from build123d import *

# Parameters (mm, degrees)
SKETCH1_W           = 24
SKETCH1_H           = 40
SKETCH2_W           = 20
SKETCH2_H           = 30
SKETCH3_W           = 20
SKETCH3_H           = 30
SKETCH4_W           = 16
SKETCH4_H           = 16
SKETCH5_W           = 11.6
SKETCH5_H           = 11.6
BOSS_EXTRUDE1_DEPTH = 10
SKETCH6_R           = 2.3
CUT_EXTRUDE1_DEPTH  = 6
SKETCH7_R           = 2.3
CUT_EXTRUDE2_DEPTH  = 6
FILLET1_R           = 1
SKETCH8_W           = 8.4
SKETCH8_H           = 24.4
CUT_EXTRUDE3_DEPTH  = 20
SKETCH9_R           = 2.3
CUT_EXTRUDE4_DEPTH  = 6


with BuildPart() as part:
    # Sketch1 → Loft1 section 0
    with BuildSketch(Plane(origin=(0, 0, 0), x_dir=(1, 0, 0), z_dir=(0, 1, 0))):
        Rectangle(SKETCH1_W, SKETCH1_H)
    # Sketch2 → Loft1 section 1
    with BuildSketch(Plane(origin=(0, 50, 0), x_dir=(1, 0, 0), z_dir=(0, 1, 0))):
        Rectangle(SKETCH2_W, SKETCH2_H)
    loft()

    # Sketch3 → Loft2 section 0
    with BuildSketch(Plane(origin=(0, 50, 0), x_dir=(1, 0, 0), z_dir=(0, 1, 0))):
        Rectangle(SKETCH3_W, SKETCH3_H)
    # Sketch4 → Loft2 section 1
    with BuildSketch(Plane(origin=(0, 76, 0), x_dir=(1, 0, 0), z_dir=(0, 1, 0))):
        Rectangle(SKETCH4_W, SKETCH4_H)
    loft()

    # Sketch5 → Boss-Extrude1 (add)
    with BuildSketch(Plane(origin=(0, 76, 0), x_dir=(1, 0, 0), z_dir=(0, 1, 0))):
        Rectangle(SKETCH5_W, SKETCH5_H)
    extrude(amount=BOSS_EXTRUDE1_DEPTH)

    # Sketch6 → Cut-Extrude1 (cut)
    with BuildSketch(Plane.XY.offset(5.8)):
        with Locations((-3, 80)):
            Circle(SKETCH6_R)
    extrude(amount=-CUT_EXTRUDE1_DEPTH, mode=Mode.SUBTRACT)

    # Sketch7 → Cut-Extrude2 (cut)
    with BuildSketch(Plane(origin=(0, 0, -5.8), x_dir=(-1, 0, 0), z_dir=(0, 0, -1))):
        with Locations((-3, 80)):
            Circle(SKETCH7_R)
    extrude(amount=-CUT_EXTRUDE2_DEPTH, mode=Mode.SUBTRACT)

    # Fillet1
    fillet1_edges = [part.edges().sort_by_distance(p)[0] for p in [
        (0, 86, 5.8),
        (5.8, 86, 0),
        (0, 86, -5.8),
        (-5.8, 86, 0),
    ]]
    fillet(fillet1_edges, radius=FILLET1_R)

    # Sketch8 → Cut-Extrude3 (cut)
    with BuildSketch(Plane.XZ):
        Rectangle(SKETCH8_W, SKETCH8_H)
    extrude(amount=-CUT_EXTRUDE3_DEPTH, mode=Mode.SUBTRACT)

    # Sketch9 → Cut-Extrude4 (cut)
    with BuildSketch(Plane.XZ):
        with Locations((0, 16)):
            Circle(SKETCH9_R)
        with Locations((0, -16)):
            Circle(SKETCH9_R)
    extrude(amount=-CUT_EXTRUDE4_DEPTH, mode=Mode.SUBTRACT)


solid = part.part
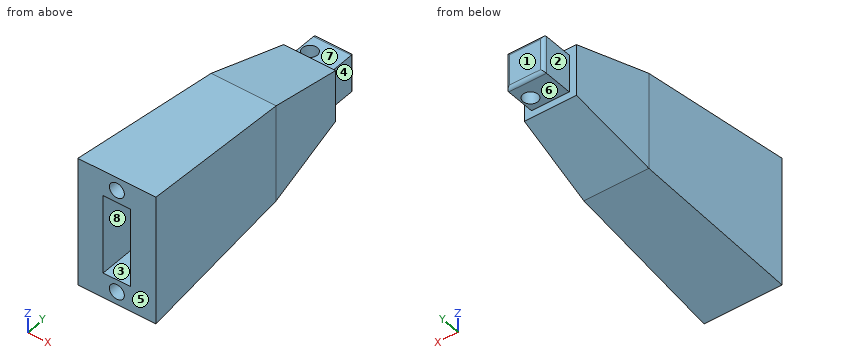
CAD build for the part. Positions are in the model's coordinates, mm. Face numbers are marked on the shaded views. A direction names the side the tool comes from. Coordinates: 2 decimals unless noted, no trailing zeros. Loops run counter-clockwise (first coordinate to the right, second up) from the corner with the lowest first, then second, coordinate; pieces in that order, holes last. Notation, with made-up numbers: (28.25, 4.5) - (40.25, 4.5) arc R12 ccw to (40.25, 10.5) - close; hole circle Ø8 at (36, 82.25). An arc over 180 degrees is marked (long way). Write item = value, one per line. Start each with the question number.
Q1. Which spindle directions (+Z, -Z, +X, -X, +Y, -Y) get a long thin tool onto all of the face, cutting with end or side? Do the marked faces 4, 5, 6, 7 and 8. Say none if no direction does.
Q2. Flat gauge pins, fed straight in: pin 1 Ø2.5 at (x, z) = (2, -5) entering from -Y; pin 2 Ø1.4 at (x, y) = (-2, 79.5) entering from +Z; pin 3 Ø4 at (x, y) = (4.5, 36.5) entering from +Z. Where does each tip first touch, or does it go through?
Q3. Cut at A-A, the plane y = 80. List the corners of the cut face in (x, z), then the cut area to 3 significant figures.
Q4. Pull direction X, two halves, no side cores. Call the marked faces 1, 2 and 3: pulls with the +X half, pulls with the -X half, needs draft (parallel to the pull), parting line crosses it, or undercut.
Q5. Drill centre lines: L1, parallel to Y at x = 3, z = -3.5; L2, parallel to Y at x = 7.25, z = -3.5; L3, parallel to Z at x = -2.5, y = 79. Where is each one in solid material? Low to high.
Computed:
q1.face_4 = +Z, -Z, +X, +Y
q1.face_5 = +Z, -Z, +X, -X, -Y
q1.face_6 = -Z, +X, -X, +Y
q1.face_7 = +Z, +X, -X, +Y
q1.face_8 = -Y
q2.pin_1 = 20
q2.pin_2 = -0.2
q2.pin_3 = 16.55
q3.outline = (-5.8, -5.8) - (0.7, -5.8) - (0.7, 0.2) - (5.3, 0.2) - (5.3, -5.8) - (5.8, -5.8) - (5.8, 5.8) - (-0.7, 5.8) - (-0.7, -0.2) - (-5.3, -0.2) - (-5.3, 5.8) - (-5.8, 5.8) - close
q3.area = 79.4 mm²
q4.face_1 = needs draft
q4.face_2 = pulls with the -X half
q4.face_3 = undercut
q5.L1 = 20 to 77.7, 82.3 to 86
q5.L2 = 0 to 76
q5.L3 = -5.8 to -0.2
